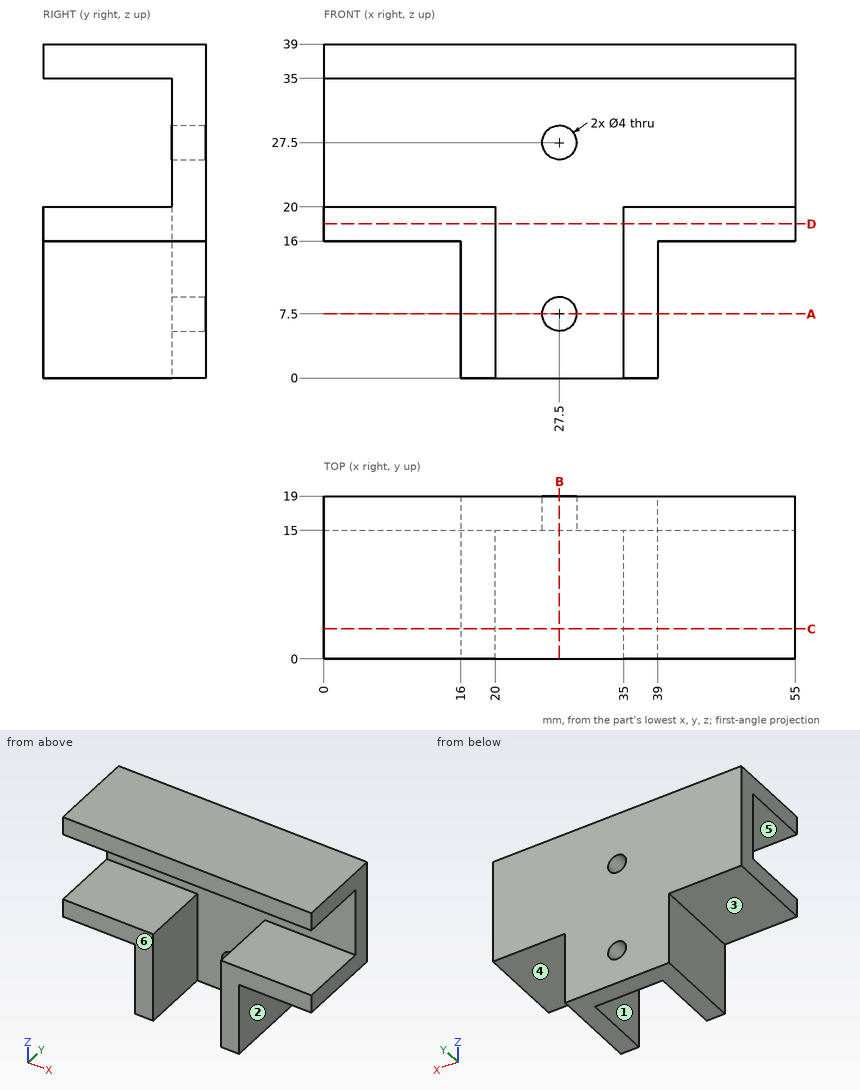
Verification items for this drawing (mm, ordinates from the low corner). A direction names the side the tool comes from. Round coordinates to 2 decimals unless told otherwise and drop trailing zeros. Order: outer loops, then holes, each group sorted by start corner. A loop starts at its lowest first (then second) coordinate and runs counter-clockwise, first axis right, second up. Notation, with made-up numbers: (32, 31.5) -> (39, 31.5) arc R20 ccw to (39, 49.5) -> close; hole circle Ø11 at (20, 44). An arc over 180 degrees is marked (long way). Use one line per item in the form item = value.
1. Set-up check for the marked faces 1, 2 and 3: record each of +Z, -Z, +X, -X, +Y, -Y from which the full face is reachable in a straight line by a thin tool's end or side.
Working result:
face_1 = -Z, -Y
face_2 = -Z, +X, +Y, -Y
face_3 = -Z, -X, +Y, -Y
2. Cross-section at C-C, the plane y = 3.5. Enter the section's corners in (x, z).
Working result:
outline = (0, 16) -> (16, 16) -> (16, 0) -> (20, 0) -> (20, 20) -> (0, 20) -> close; (0, 35) -> (55, 35) -> (55, 39) -> (0, 39) -> close; (35, 0) -> (39, 0) -> (39, 16) -> (55, 16) -> (55, 20) -> (35, 20) -> close
3. Go/stop test with flat-tipped pins: pin 1 (8 mm diameter, centred on y = 10.5, z = 5, fed in from +X); pin 2 (2.5 mm diameter, centred on x = 27.5, z = 7.5, fed in from -Y); pin 3 (5 mm diameter, centred on x = 45, y = 8, fed in from -Z); pin 4 (4.5 mm diameter, centred on y = 9.5, z = 8, fed in from -X). Record where each tip stops, or that it passes through.
Working result:
pin_1 = 39
pin_2 = through
pin_3 = 16
pin_4 = 16
4. Mould release check, pull along Z, two halves, no side actions. Record for the marked faces 4, 5 and 6: pulls with the +Z half, pulls with the -Z half, needs draft (parallel to the pull), parting line crosses it, or undercut.
Working result:
face_4 = pulls with the -Z half
face_5 = undercut
face_6 = needs draft
5. Cross-section at B-B, the plane x = 27.5. Enter the section's corners in (y, z), plus the area to 3 significant figures.
Working result:
outline = (0, 35) -> (15, 35) -> (15, 29.5) -> (19, 29.5) -> (19, 39) -> (0, 39) -> close; (15, 0) -> (19, 0) -> (19, 5.5) -> (15, 5.5) -> close; (15, 9.5) -> (19, 9.5) -> (19, 25.5) -> (15, 25.5) -> close
area = 184 mm^2
6. Cross-section at A-A, the plane z = 7.5. Enter the section's corners in (x, y).
Working result:
outline = (16, 0) -> (20, 0) -> (20, 15) -> (25.5, 15) -> (25.5, 19) -> (16, 19) -> close; (29.5, 15) -> (35, 15) -> (35, 0) -> (39, 0) -> (39, 19) -> (29.5, 19) -> close
7. Scan lines: line 1 along Z through (x, y) = (27.5, 17.9); line 2 along Z through (x, y) = (4.5, 6); line 3 along Z through (x, y) = (19.5, 3). Record each from-to range of solid material in increasing order. Write a range as from..to.
Working result:
line_1 = 0..5.5, 9.5..25.5, 29.5..39
line_2 = 16..20, 35..39
line_3 = 0..20, 35..39
8. Cross-section at D-D, the plane z = 18. Enter the section's corners in (x, y).
Working result:
outline = (0, 0) -> (20, 0) -> (20, 15) -> (35, 15) -> (35, 0) -> (55, 0) -> (55, 19) -> (0, 19) -> close
